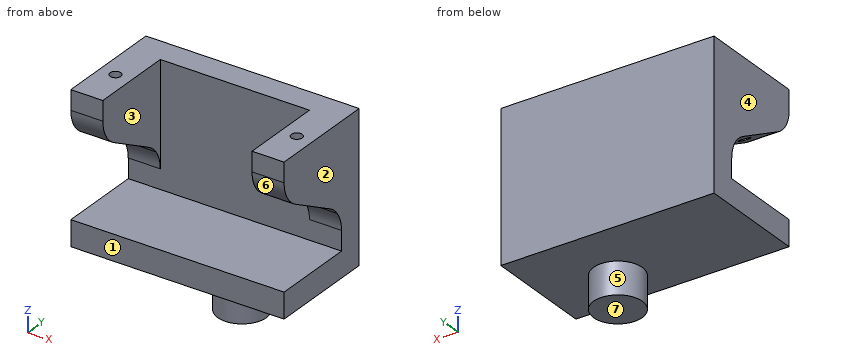
from build123d import *

# Parameters (mm, degrees)
F1_W     = 5
F1_H     = 7.2
F1_H_2   = 6
F1_H_3   = 4
F1_W_2   = 23.3
F3_DEPTH = 8.5
F4_DEPTH = 23.2
F5_DEPTH = 18.1
F6_START = 4.3
F0_R     = 0.85
F6_DEPTH = 20.7
F0_R_2   = 3.8
F7_DEPTH = 5


with BuildPart() as f3:
    # F1 (on Front) → F3 (new body, symmetric)
    with BuildSketch(Plane.XZ):
        with Locations((-14.15, 13.6)):
            Rectangle(F1_W, F1_H)
        with Locations((-14.15, 20.2)):
            Rectangle(F1_W, F1_H_2)
        with Locations((-14.15, 7)):
            Rectangle(F1_W, F1_H_2)
        with Locations((-14.15, 2)):
            Rectangle(F1_W, F1_H_3)
        with Locations((0, 2)):
            Rectangle(F1_W_2, F1_H_3)
        with Locations((14.15, 2)):
            Rectangle(F1_W, F1_H_3)
        with Locations((14.15, 7)):
            Rectangle(F1_W, F1_H_2)
        with Locations((14.15, 13.6)):
            Rectangle(F1_W, F1_H)
        with Locations((14.15, 20.2)):
            Rectangle(F1_W, F1_H_2)
    extrude(amount=F3_DEPTH, both=True)

    # F0 (on Top) → F4 (join)
    with BuildSketch(Plane.XY):
        Polygon((11.65, 4.5), (11.65, 8.5), (0, 8.5), (-11.65, 8.5), (-11.65, 4.5), align=None)
    extrude(amount=F4_DEPTH)

    # F2 (on Right) → F5 (cut, symmetric)
    with BuildSketch(Plane.YZ):
        with BuildLine():
            Line((-8.5, 17.2), (-8.5, 10))
            Line((-8.5, 10), (3.5396314061, 10))
            ThreePointArc((3.5396314061, 10), (2.8089650426, 10.8020152096), (1.9224991399, 11.4275389379))
            Line((1.9224991399, 11.4275389379), (-5.9224991399, 15.7724610621))
            ThreePointArc((-5.9224991399, 15.7724610621), (-6.8089650426, 16.3979847904), (-7.5396314061, 17.2))
            Line((-7.5396314061, 17.2), (-8.5, 17.2))
        make_face()
        with BuildLine():
            Line((-8.5, 20.1464178425), (-8.5, 17.2))
            Line((-8.5, 17.2), (-7.5396314061, 17.2))
            ThreePointArc((-7.5396314061, 17.2), (-8.2538488107, 18.5969271247), (-8.5, 20.1464178425))
        make_face()
        with BuildLine():
            Line((-8.5, 10), (-8.5, 4))
            Line((-8.5, 4), (4.5, 4))
            Line((4.5, 4), (4.5, 7.0535821575))
            ThreePointArc((4.5, 7.0535821575), (4.2538488107, 8.6030728753), (3.5396314061, 10))
            Line((3.5396314061, 10), (-8.5, 10))
        make_face()
    extrude(amount=F5_DEPTH, both=True, mode=Mode.SUBTRACT)

    # F0 (on Top) → F6 (cut)
    with BuildSketch(Plane.XY.offset(F6_START)):
        with Locations((14.15, -2)):
            Circle(F0_R)
        with Locations((-14.15, -2)):
            Circle(F0_R)
    extrude(amount=F6_DEPTH, mode=Mode.SUBTRACT)

    # F0 (on Top) → F7 (join)
    with BuildSketch(Plane.XY):
        with Locations((5.75, -2.2)):
            Circle(F0_R_2)
    extrude(amount=-F7_DEPTH)


solid = f3.part
Could you check a few things on this model? Use its own coordinates, in mm. Face numbers are marked on the shaded views. A direction names the side the tool comes from. Give positions to 0.01 mm unless a question says otherwise; leave off trailing zeros. Order: outer loops, then holes, each group sorted by start corner. A loop starts at its lowest first (then second) coordinate and runs counter-clockwise, first axis right, second up.
Item 1: I'm going to push flat-ended pins straight in: pin 1 (6.5 mm diameter, centred on x = 0.5, y = -4.5, fed in from +Z); pin 2 (5 mm diameter, centred on x = 2.5, y = 4, fed in from -Z); pin 3 (15.5 mm diameter, centred on x = 1, z = 14, fed in from -Y). Where does each tip first touch, or does it pass through?
Item 2: If we mould it in two halves opening along X, with no side actions, what happens to the marked faces 1, 2, 3 and 4? For each: pulls with the +X half, pulls with the -X half, needs draft (parallel to the pull), parting line crosses it, or undercut.
Item 3: For the marked faces 5, 6 and 7, which set-ups out of +Z, -Z, +X, -X, +Y, -Y let a thin tool reach every point of the face, with its end or its side?
Item 4: If we section it at D-D, the plane y = 4: Write out the boundary of the cut face in (x, z).
Item 5: If we section it at C-C, the plane x = 14.5: Write out the boundary of the cut face in (y, z), plus the area to 3 significant figures.
Item 6: If we section it at B-B, the plane x = 5.75: Write out the boundary of the cut face in (y, z).
Item 7: I need wall thicknesses on line 1 (X direction, y = -2, z = 18.25); line 2 (Y direction, x = 1, z = 7.25); line 3 (Z direction, x = 15, y = 6). Which ranges of each line are inside material? Lowest first, please.
Item 8: If we section it at A-A, the plane z = 21.25: Write out the boundary of the cut face in (x, y).
Values:
1. pin 1: stops at z = 4
1. pin 2: stops at z = 0
1. pin 3: stops at y = 4.5
2. face 1: needs draft
2. face 2: pulls with the +X half
2. face 3: undercut
2. face 4: pulls with the -X half
3. face 5: -Z
3. face 6: +X, -X, -Y
3. face 7: -Z, +X, -X, +Y, -Y
4. outline: (-16.65, 0) - (16.65, 0) - (16.65, 4) - (-16.65, 4) - close; (-16.65, 9.23) - (-11.65, 9.23) - (-11.65, 23.2) - (-16.65, 23.2) - close; (11.65, 9.23) - (16.65, 9.23) - (16.65, 23.2) - (11.65, 23.2) - close
5. outline: (-8.5, 0) - (8.5, 0) - (8.5, 23.2) - (-1.23, 23.2) - (-1.23, 13.17) - (1.92, 11.43) arc R5 cw to (4.5, 7.05) - (4.5, 4) - (-8.5, 4) - close; (-8.5, 20.15) arc R5 ccw to (-5.92, 15.77) - (-2.77, 14.03) - (-2.77, 23.2) - (-8.5, 23.2) - close
5. area: 255 mm2
6. outline: (-8.5, 0) - (-6, 0) - (-6, -5) - (1.6, -5) - (1.6, 0) - (8.5, 0) - (8.5, 23.2) - (4.5, 23.2) - (4.5, 4) - (-8.5, 4) - close
7. line 1: x = -16.65 to -15, -13.3 to -11.65, 11.65 to 13.3, 15 to 16.65
7. line 2: y = 4.5 to 8.5
7. line 3: z = 0 to 23.2
8. outline: (-16.65, -8.5) - (-11.65, -8.5) - (-11.65, 4.5) - (11.65, 4.5) - (11.65, -8.5) - (16.65, -8.5) - (16.65, 8.5) - (-16.65, 8.5) - close; hole circle Ø1.7 at (-14.15, -2); hole circle Ø1.7 at (14.15, -2)
